The model under review builds one solid part; all positions refer to its coordinate system, in mm. Face numbers are marked on the shaded views. Give positions to 0.01 mm unless a question says otherwise; leave off trailing zeros. Answer as CSV lines item,"result". Start each with the question number.
from build123d import *

# Parameters (mm, degrees)
SKETCH_1_W      = 4
SKETCH_1_H      = 6
EXTRUDE_1_DEPTH = 10
EXTRUDE_2_DEPTH = 20
SKETCH_1_4_W    = 4
SKETCH_1_4_H    = 6
EXTRUDE_3_DEPTH = 10
FILLET_1_R      = 5
EXTRUDE_4_DEPTH = 25
EXTRUDE_START   = 25
EXTRUDE_5_DEPTH = 5
EXTRUDE_START_2 = -25
EXTRUDE_6_DEPTH = 5
EXTRUDE_START_3 = 15
EXTRUDE_7_DEPTH = 10
EXTRUDE_8_DEPTH = 10
FILLET_2_R      = 5


with BuildPart() as part:
    # Sketch 1 → Extrude 1 (new body)
    with BuildSketch(Plane(origin=(0, 0, 0), x_dir=(1, 0, 0), z_dir=(0, 1, 0))):
        with BuildLine():
            Line((-200, -100), (200, -100))
            ThreePointArc((200, -100), (300, 0), (200, 100))
            Line((200, 100), (-200, 100))
            ThreePointArc((-200, 100), (-300, 0), (-200, -100))
        make_face()
        with Locations((-242, 18)):
            Rectangle(SKETCH_1_W, SKETCH_1_H, mode=Mode.SUBTRACT)
        with Locations((-242, -18)):
            Rectangle(SKETCH_1_W, SKETCH_1_H, mode=Mode.SUBTRACT)
    extrude(amount=EXTRUDE_1_DEPTH)

    # Sketch 1_3 → Extrude 2 (add)
    with BuildSketch(Plane(origin=(0, 0, 0), x_dir=(1, 0, 0), z_dir=(0, 1, 0))):
        with BuildLine():
            Line((-200, 110), (200, 110))
            ThreePointArc((200, 110), (310, 0), (200, -110))
            Line((200, -110), (-200, -110))
            ThreePointArc((-200, -110), (-310, 0), (-200, 110))
        make_face()
        with BuildLine():
            ThreePointArc((200, -100), (300, 0), (200, 100))
            Line((200, 100), (-200, 100))
            ThreePointArc((-200, 100), (-300, 0), (-200, -100))
            Line((-200, -100), (200, -100))
        make_face(mode=Mode.SUBTRACT)
    extrude(amount=EXTRUDE_2_DEPTH)

    # Sketch 1_4 → Extrude 3 (add)
    with BuildSketch(Plane(origin=(0, 0, 0), x_dir=(1, 0, 0), z_dir=(0, 1, 0))):
        with Locations((-242, 18)):
            Rectangle(SKETCH_1_4_W, SKETCH_1_4_H)
        with Locations((-242, -18)):
            Rectangle(SKETCH_1_4_W, SKETCH_1_4_H)
    extrude(amount=EXTRUDE_3_DEPTH)

    # Fillet 1
    fillet_1_edges = [part.edges().sort_by_distance(p)[0] for p in [
        (0, 20, -110),
        (300, 20, 0),
        (0, 20, 100),
        (-300, 20, 0),
        (0, 20, -100),
        (-310, 20, 0),
        (0, 20, 110),
        (310, 20, 0),
    ]]
    fillet(fillet_1_edges, radius=FILLET_1_R - 0.0001)  # a hair under: the kernel refuses the full size



with BuildPart() as body_2:
    # Sketch 2 → Extrude 4 (new, symmetric)
    with BuildSketch(Plane.XY):
        with BuildLine():
            ThreePointArc((-245, 230), (-256.715728753, 258.284271247), (-285, 270))
            Line((-285, 270), (-325, 270))
            Line((-325, 270), (-325, 265))
            Line((-325, 265), (-285, 265))
            ThreePointArc((-285, 265), (-260.251262658, 254.748737342), (-250, 230))
            ThreePointArc((-250, 230), (-247.484567313, 197.984378813), (-240, 166.754446797))
            ThreePointArc((-240, 166.754446797), (-235.413108769, 154.053650458), (-230, 141.682391337))
            ThreePointArc((-230, 141.682391337), (-172.840678712, 69.744700973), (-90, 30))
            ThreePointArc((-90, 30), (-85.012374627, 28.942769648), (-80, 28.009901233))
            ThreePointArc((-80, 28.009901233), (-66.253520421, 26.104713469), (-52.409638554, 25.133952895))
            ThreePointArc((-52.409638554, 25.133952895), (-50.700569032, 24.371111803), (-50, 22.635586467))
            Line((-50, 22.635586467), (-45, 22.635586467))
            ThreePointArc((-45, 22.635586467), (-47.101707097, 27.842162475), (-52.228915663, 30.130685751))
            ThreePointArc((-52.228915663, 30.130685751), (-188.95447741, 91.1579731), (-245, 230))
        make_face()
    extrude(amount=EXTRUDE_4_DEPTH, both=True)


with BuildPart() as body_3:
    # Sketch 2_4 → Extrude 5 (new body)
    with BuildSketch(Plane.XY.offset(EXTRUDE_START)):
        with BuildLine():
            Line((-325, 270), (-285, 270))
            ThreePointArc((-285, 270), (-256.715728753, 258.284271247), (-245, 230))
            ThreePointArc((-245, 230), (-188.95447741, 91.1579731), (-52.228915663, 30.130685751))
            ThreePointArc((-52.228915663, 30.130685751), (-47.101707097, 27.842162475), (-45, 22.635586467))
            Line((-45, 22.635586467), (-40, 22.635586467))
            ThreePointArc((-40, 22.635586467), (-43.502845162, 31.313213148), (-52.048192771, 35.127418607))
            ThreePointArc((-52.048192771, 35.127418607), (-185.355615474, 94.629023772), (-240, 230))
            ThreePointArc((-240, 230), (-253.180194847, 261.819805153), (-285, 275))
            Line((-285, 275), (-325, 275))
            Line((-325, 275), (-325, 270))
        make_face()
    extrude(amount=-EXTRUDE_5_DEPTH)


with BuildPart() as body_4:
    # Sketch 2_5 → Extrude 6 (new body)
    with BuildSketch(Plane.XY.offset(EXTRUDE_START_2)):
        with BuildLine():
            Line((-325, 270), (-285, 270))
            ThreePointArc((-285, 270), (-256.715728753, 258.284271247), (-245, 230))
            ThreePointArc((-245, 230), (-188.95447741, 91.1579731), (-52.228915663, 30.130685751))
            ThreePointArc((-52.228915663, 30.130685751), (-47.101707097, 27.842162475), (-45, 22.635586467))
            Line((-45, 22.635586467), (-40, 22.635586467))
            ThreePointArc((-40, 22.635586467), (-43.502845162, 31.313213148), (-52.048192771, 35.127418607))
            ThreePointArc((-52.048192771, 35.127418607), (-185.355615474, 94.629023772), (-240, 230))
            ThreePointArc((-240, 230), (-253.180194847, 261.819805153), (-285, 275))
            Line((-285, 275), (-325, 275))
            Line((-325, 275), (-325, 270))
        make_face()
    extrude(amount=EXTRUDE_6_DEPTH)



with BuildPart() as part_1:
    add(part.part)

    add(body_2.part)  # Extrude 7 merges body 2

    add(body_3.part)  # Extrude 7 merges body 3
    # Sketch 2_8 → Extrude 7 (add)
    with BuildSketch(Plane.XY.offset(EXTRUDE_START_3)):
        with BuildLine():
            ThreePointArc((-230, 141.682391337), (-235.413108769, 154.053650458), (-240, 166.754446797))
            Line((-240, 166.754446797), (-240, 0))
            Line((-240, 0), (-230, 0))
            Line((-230, 0), (-230, 141.682391337))
        make_face()
        with BuildLine():
            Line((-80, 0), (-80, 28.009901233))
            ThreePointArc((-80, 28.009901233), (-85.012374627, 28.942769648), (-90, 30))
            Line((-90, 30), (-90, 0))
            Line((-90, 0), (-80, 0))
        make_face()
    extrude(amount=EXTRUDE_7_DEPTH)


with BuildPart() as body_4_1:
    add(body_4.part)

    add(part_1.part)  # Extrude 8 merges part
    # Sketch 2_9 → Extrude 8 (add)
    with BuildSketch(Plane.XY.offset(EXTRUDE_START_2)):
        with BuildLine():
            ThreePointArc((-230, 141.682391337), (-235.413108769, 154.053650458), (-240, 166.754446797))
            Line((-240, 166.754446797), (-240, 0))
            Line((-240, 0), (-230, 0))
            Line((-230, 0), (-230, 141.682391337))
        make_face()
        with BuildLine():
            Line((-80, 0), (-80, 28.009901233))
            ThreePointArc((-80, 28.009901233), (-85.012374627, 28.942769648), (-90, 30))
            Line((-90, 30), (-90, 0))
            Line((-90, 0), (-80, 0))
        make_face()
    extrude(amount=EXTRUDE_8_DEPTH)

    # Fillet 2
    fillet_2_edges = [body_4_1.edges().sort_by_distance(p)[0] for p in [
        (-305, 275, -25),
        (-253.180194847, 261.819805153, -25),
        (-43.502845162, 31.313213148, -25),
        (-305, 275, 25),
        (-253.180194847, 261.819805153, 25),
        (-43.502845162, 31.313213148, 25),
        (-185.355615474, 94.629023772, -25),
        (-185.355615474, 94.629023772, 25),
    ]]
    fillet(fillet_2_edges, radius=FILLET_2_R - 0.0001)  # a hair under: the kernel refuses the full size


solid = body_4_1.part
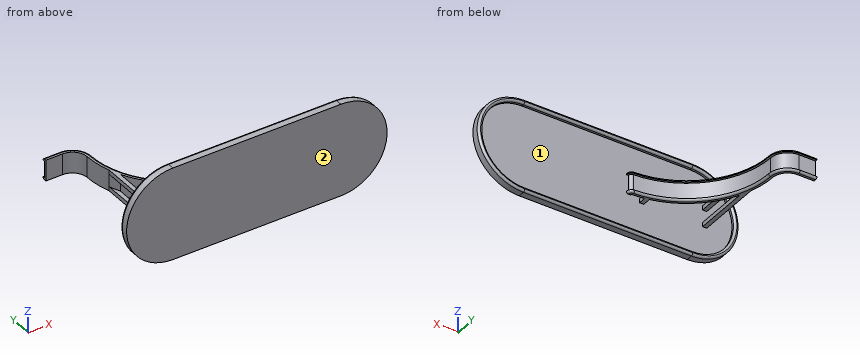
Item 1: Clearance check with flat-ended pins moving along their axes: pin 1 (1.5 mm diameter, centred on x = -157.5, z = -26, fed in from +Y); pin 2 (11 mm diameter, centred on y = 15, z = 21, fed in from +X); pin 3 (5 mm diameter, centred on x = -46.5, z = -12.5, fed in from -Y); pin 4 (3 mm diameter, centred on x = -83, y = 24, fed in from -Z). State where each tip first meets the part, or that it passes through.
Item 2: Mouldability with a two-part tool opening along Z and no side actions: class the marked faces 1 and 2 as released by +Z, released by -Z, zero draft, split by the parting line, or undercut.
Item 3: For line 1 along Z through (x, y) = (135.5, 15.5); line 2 along Y through (x, z) = (-166, -29.5); line 3 along Y through (x, z) = (-188, -11), list the stretches that pass through material, from the lowest coordinate up.
Item 4: Take a section at B-B on y = 88.5. Count the separate pieces of the cut face and the enclosed holes in it, and give its area (3 significant figures).
Data:
1,pin 1,"stops at y = 10"
1,pin 2,"stops at x = 308.9"
1,pin 3,"stops at y = 0"
1,pin 4,"stops at z = -25"
2,face 1,"undercut"
2,face 2,"zero draft"
3,line 1,"z = -109.97 to -100.03, 100.03 to 109.97"
3,line 2,"y = 0 to 10"
3,line 3,"y = 0 to 10, 83.11 to 90.18"
4,separate pieces,"3"
4,enclosed holes,"0"
4,area,"606 mm^2"
